from build123d import *

# Parameters (mm, degrees)
SKETCH1_W          = 155
SKETCH1_H          = 498.5268
BASE_FLANGE1_DEPTH = 5
CUT_EXTRUDE2_REACH = 473.277
SKETCH6_R          = 7.5
CUT_EXTRUDE3_REACH = 473.277
SKETCH7_R          = 4
FILLET1_R          = 10


# Sheet-metal steps are written as plain solids
with BuildPart() as part:
    # Sketch1 → Base-Flange1 (new body)
    with BuildSketch(Plane.XY):
        with Locations((-77.5, -195.767163373)):
            Rectangle(SKETCH1_W, SKETCH1_H)
    extrude(amount=BASE_FLANGE1_DEPTH)

    # Sketch6 → Cut-Extrude2 (cut, up to next)
    with BuildSketch(Plane.XY.offset(5), mode=Mode.PRIVATE) as cut_extrude2_sk1:
        with Locations((-77.5, -367.367664241)):
            Circle(SKETCH6_R)
    cut_extrude2_tool1 = extrude(cut_extrude2_sk1.sketch, amount=-CUT_EXTRUDE2_REACH, mode=Mode.PRIVATE) & part.part
    # Sketch6 → Cut-Extrude2 (cut, up to next)
    with BuildSketch(Plane.XY.offset(5), mode=Mode.PRIVATE) as cut_extrude2_sk2:
        with Locations((-77.5, -29.166662504)):
            Circle(SKETCH6_R)
    cut_extrude2_tool2 = extrude(cut_extrude2_sk2.sketch, amount=-CUT_EXTRUDE2_REACH, mode=Mode.PRIVATE) & part.part
    add(cut_extrude2_tool1.solids().sort_by_distance((-77.5, -367.367664, 5))[0], mode=Mode.SUBTRACT)
    add(cut_extrude2_tool2.solids().sort_by_distance((-77.5, -29.166663, 5))[0], mode=Mode.SUBTRACT)

    # Sketch7 → Cut-Extrude3 (cut, up to next)
    with BuildSketch(Plane.XY.offset(5), mode=Mode.PRIVATE) as cut_extrude3_sk1:
        with Locations((-110.070394878, -433.005563373)):
            Circle(SKETCH7_R)
    cut_extrude3_tool1 = extrude(cut_extrude3_sk1.sketch, amount=-CUT_EXTRUDE3_REACH, mode=Mode.PRIVATE) & part.part
    # Sketch7 → Cut-Extrude3 (cut, up to next)
    with BuildSketch(Plane.XY.offset(5), mode=Mode.PRIVATE) as cut_extrude3_sk2:
        with Locations((-75.272394878, -433.005563373)):
            Circle(SKETCH7_R)
    cut_extrude3_tool2 = extrude(cut_extrude3_sk2.sketch, amount=-CUT_EXTRUDE3_REACH, mode=Mode.PRIVATE) & part.part
    # Sketch7 → Cut-Extrude3 (cut, up to next)
    with BuildSketch(Plane.XY.offset(5), mode=Mode.PRIVATE) as cut_extrude3_sk3:
        with Locations((-40.474394878, -433.005563373)):
            Circle(SKETCH7_R)
    cut_extrude3_tool3 = extrude(cut_extrude3_sk3.sketch, amount=-CUT_EXTRUDE3_REACH, mode=Mode.PRIVATE) & part.part
    # Sketch7 → Cut-Extrude3 (cut, up to next)
    with BuildSketch(Plane.XY.offset(5), mode=Mode.PRIVATE) as cut_extrude3_sk4:
        with Locations((-42.712394878, 41.471236627)):
            Circle(SKETCH7_R)
    cut_extrude3_tool4 = extrude(cut_extrude3_sk4.sketch, amount=-CUT_EXTRUDE3_REACH, mode=Mode.PRIVATE) & part.part
    # Sketch7 → Cut-Extrude3 (cut, up to next)
    with BuildSketch(Plane.XY.offset(5), mode=Mode.PRIVATE) as cut_extrude3_sk5:
        with Locations((-76.748394878, 41.471236627)):
            Circle(SKETCH7_R)
    cut_extrude3_tool5 = extrude(cut_extrude3_sk5.sketch, amount=-CUT_EXTRUDE3_REACH, mode=Mode.PRIVATE) & part.part
    # Sketch7 → Cut-Extrude3 (cut, up to next)
    with BuildSketch(Plane.XY.offset(5), mode=Mode.PRIVATE) as cut_extrude3_sk6:
        with Locations((-110.784394878, 41.471236627)):
            Circle(SKETCH7_R)
    cut_extrude3_tool6 = extrude(cut_extrude3_sk6.sketch, amount=-CUT_EXTRUDE3_REACH, mode=Mode.PRIVATE) & part.part
    add(cut_extrude3_tool1.solids().sort_by_distance((-110.070395, -433.005563, 5))[0], mode=Mode.SUBTRACT)
    add(cut_extrude3_tool2.solids().sort_by_distance((-75.272395, -433.005563, 5))[0], mode=Mode.SUBTRACT)
    add(cut_extrude3_tool3.solids().sort_by_distance((-40.474395, -433.005563, 5))[0], mode=Mode.SUBTRACT)
    add(cut_extrude3_tool4.solids().sort_by_distance((-42.712395, 41.471237, 5))[0], mode=Mode.SUBTRACT)
    add(cut_extrude3_tool5.solids().sort_by_distance((-76.748395, 41.471237, 5))[0], mode=Mode.SUBTRACT)
    add(cut_extrude3_tool6.solids().sort_by_distance((-110.784395, 41.471237, 5))[0], mode=Mode.SUBTRACT)

    # Fillet1
    # the kernel refuses this fillet: 10 mm, written as the material it takes off along each edge
    with BuildSketch(Plane(origin=(-155, 75.146871722, 5), x_dir=(0, 0, -1), z_dir=(0, -1, 0))) as fillet1_piece_1:
        with BuildLine():
            CenterArc((10, 8.660254038), FILLET1_R, 180, 60)
            Line((0, 8.660254038), (-0.2, 8.660254038))
            Line((-0.2, 8.660254038), (-0.2, 0))
            Line((-0.2, 0), (0, -0.2))
            ThreePointArc((0, -0.2), (2.5, -0.2), (4.9, -0.173205081))
            Line((4.9, -0.173205081), (5, 0))
        make_face()
    extrude(amount=541.828070189, mode=Mode.SUBTRACT)


solid = part.part
Work out the finished part from the listing and answer in its coordinate system (mm). Round coordinates to 2 decimals unless told otherwise and drop trailing zeros. Write each loop counter-clockwise with the first axis right and the second up, starting at its lowest first coordinate (ties: lowest second). Pieces come first, ordered by that corner, then holes. Notation, with made-up numbers: (-36, 29) - (-10, 29) arc R18 cw to (-10, 47) - close; hole circle Ø8 at (75, 82.5). An arc over 180 degrees is marked (long way). Answer in a Markdown table with one row per item. Add a question column.
1. Find the intervals of material crossed by line 1 along Y through (x, z) = (-76.5, 4.1); line 2 along Y through (x, z) = (-109, 4.35); line 3 along X through (y, z) = (-210.5, 3.65), in increasing order. Write a range as from..to.
2. A cutting plane is placed at A-A, the plane z = 1.8. Count the separate pieces of the cut face and the enclosed holes in it, and give its area (3 significant figures).
3. The mould has two halves that part along X. Classify faces 1 (the cylindrical face through (-151.276, -192.277, 3.697)), 2 (the flat face through (-79, -192, 0)), 3 (the cylindrical face through (-110.94, -436.91, 2.54)), 4 (the cylindrical face through (-80.745, 41.647, 2.535)): +X half, -X half, draft (parallel to the pull), parting line (faces both ways), or undercut.
4. A cutting plane is placed at B-B, the plane y = 8. Determine the outline of the cut face in (x, z).
5. Given pin 1 (1.5 mm diameter, centred on x = -23.5, y = -392, fed in from -Z); pin 2 (2 mm diameter, centred on y = -44, z = 4, fed in from -X), each flat-ended and moving along its own axis, determine where each tip first touches the part or whether it passes through.
Worked out:
| question | item | result |
|---|---|---|
| 1 | line 1 | -445.03..-436.81, -429.2..-374.8, -359.93..-36.6, -21.73..37.48, 45.46..53.5 |
| 1 | line 2 | -445.03..-436.86, -429.15..37.89, 45.05..53.5 |
| 1 | line 3 | -151.36..0 |
| 2 | separate pieces | 1 |
| 2 | enclosed holes | 8 |
| 2 | area | 76,000 mm^2 |
| 3 | face 1 | -X half |
| 3 | face 2 | draft |
| 3 | face 3 | undercut |
| 3 | face 4 | undercut |
| 4 | outline | (-155, 0) - (0, 0) - (0, 5) - (-146.34, 5) arc R10 ccw to start |
| 5 | pin 1 | z = 0 |
| 5 | pin 2 | x = -152.34 |
